Verification items for this drawing (mm, ordinates from the low corner). A direction names the side the tool comes from. Give positions to 0.01 mm unless a question says otherwise; leave off trailing zeros. Write each loop counter-clockwise with the first axis right and the second up, starting at its lowest first coordinate (ties: lowest second). Pieces come first, ordered by that corner, then holes. Notation, with made-up numbers: (77.25, 2.25) -> (120.25, 2.25) arc R18 ccw to (120.25, 18.25) -> close; hole circle Ø10 at (-14, 50.5). An arc over 180 degrees is marked (long way). Use one line per item in the form item = value. Start each with the question number.
(1) Section check C-C, the plane y = 11.5. Record the cut outline in (x, z) (3 decimals), plus the area to 3 significant figures.
(2) Scan lines: L1, parallel to Y at x = 22, z = 35; L2, parallel to X at y = 16.5, z = 21; L3, parallel to X at y = 32, z = 20.5. Record each from-to range of solid material in increasing order.
(3) Set-up check for the marked faces 4 and 5: record each of +Z, -Z, +X, -X, +Y, -Y from which the full face is reachable in a straight line by a thin tool's end or side.
(4) Section check B-B, the plane y = 33. Record the cut outline in (x, z) (3 decimals), plus the area to 3 significant figures.
(5) Section check A-A, the plane z = 20. Record the cut outline in (x, y).
(6) Depth check by flat-ended pin: pin 1 Ø3 at (x, y) = (33, 34.5) entering from +Z; pin 2 Ø3 at (y, z) = (8, 17) entering from +X; pin 3 Ø1 at (x, y) = (32, 32.5) entering from -Z; pin 4 Ø1.5 at (x, z) = (35, 4) entering from -Y. Enter the tip coordinate at first touch or a pass-through.
(7) Release check for a two-part mould opening along X. For the marked faces 1, 2 and 3 record: pulls with the +X half, pulls with the -X half, needs draft (parallel to the pull), parting line crosses it, or undercut.
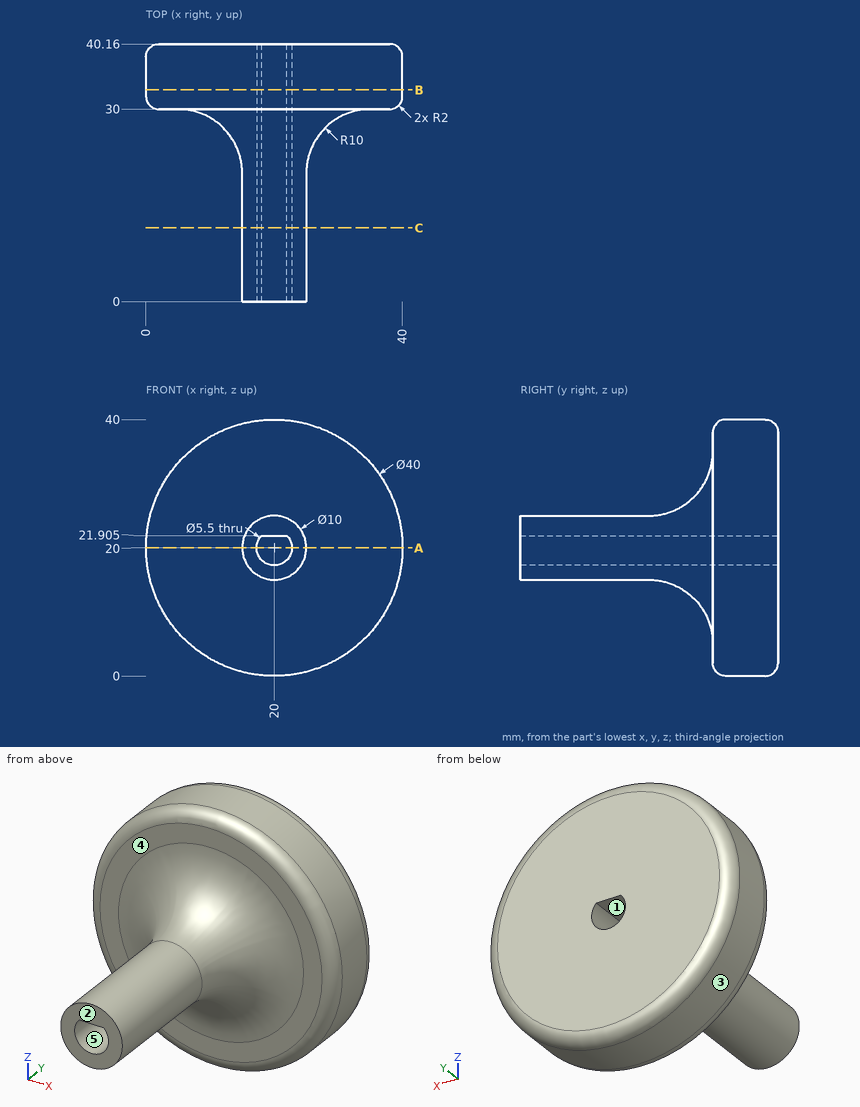
Completed:
q1.outline = circle Ø10 at (20, 20); hole (18.017, 21.905) arc R2.75 ccw (long way) to (21.983, 21.905) -> close
q1.area = 57.1 mm²
q2.L1 = 30 to 40.16
q2.L2 = 15.1 to 17.44, 22.56 to 24.9
q2.L3 = 0.01 to 17.3, 22.7 to 39.99
q3.face_4 = -Y
q3.face_5 = +Y, -Y
q4.outline = circle Ø40 at (20, 20); hole (18.017, 21.905) arc R2.75 ccw (long way) to (21.983, 21.905) -> close
q4.area = 1,240 mm²
q5.outline = (0, 32) arc R2 ccw to (2, 30) -> (5, 30) arc R10 cw to (15, 20) -> (15, 0) -> (17.25, 0) -> (17.25, 40.16) -> (2, 40.16) arc R2 ccw to (0, 38.16) -> close; (22.75, 0) -> (25, 0) -> (25, 20) arc R10 cw to (35, 30) -> (38, 30) arc R2 ccw to (40, 32) -> (40, 38.16) arc R2 ccw to (38, 40.16) -> (22.75, 40.16) -> close
q6.pin_1 = 36.36
q6.pin_2 = 24.77
q6.pin_3 = 3.64
q6.pin_4 = through
q7.face_1 = undercut
q7.face_2 = needs draft
q7.face_3 = parting line crosses it
